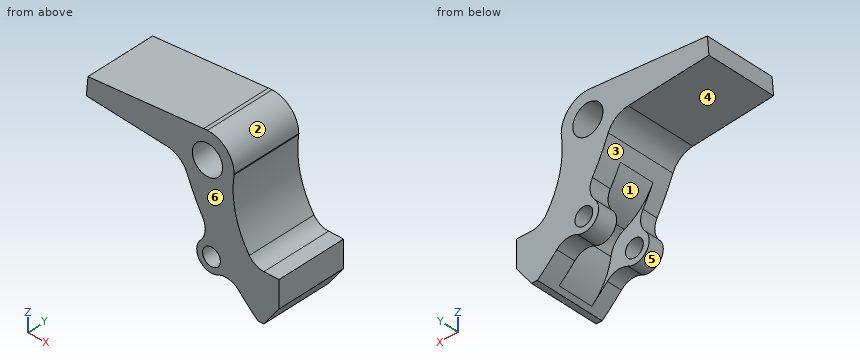
```python
from build123d import *

# Parameters (mm, degrees)
SKETCH1_R           = 2.55
SKETCH1_R_2         = 1.5
BOSS_EXTRUDE1_DEPTH = 11.9
SKETCH2_R           = 4
CUT_EXTRUDE1_DEPTH  = 3
FILLET1_R           = 10


with BuildPart() as part:
    # Sketch1 → Boss-Extrude1 (new body)
    with BuildSketch(Plane(origin=(0, 0, 0), x_dir=(1, 0, 0), z_dir=(0, 1, 0))):
        with BuildLine():
            Line((9.548719517, 20.446351577), (8.548719517, 20.439520648))
            ThreePointArc((8.548719517, 20.439520648), (6.873073378, 18.92667054), (5.279413844, 17.32768501))
            ThreePointArc((5.279413844, 17.32768501), (3.641729047, 16.438171118), (1.79479604, 16.687339585))
            ThreePointArc((1.79479604, 16.687339585), (-1.298720161, 15.927784086), (-1.135127046, 12.74658866))
            ThreePointArc((-1.135127046, 12.74658866), (-0.36458096, 11.049678177), (-0.744733852, 9.225197364))
            ThreePointArc((-0.744733852, 9.225197364), (-2.181853542, 6.500169129), (-3.4195031, 3.678943251))
            ThreePointArc((-3.4195031, 3.678943251), (-4.750151746, 1.944049699), (-6.794216917, 1.167983317))
            Line((-6.794216917, 1.167983317), (-20.434932532, -0.008444123))
            Line((-20.434932532, -0.008444123), (-20.171389856, -3.064230295))
            Line((-20.171389856, -3.064230295), (-0.61568325, -4.46265538))
            Line((-0.61568325, -4.46265538), (0.024630797, -4.508444123))
            ThreePointArc((0.024630797, -4.508444123), (3.206611312, -3.190424639), (4.524630797, -0.008444123))
            ThreePointArc((4.524630797, -0.008444123), (4.522964187, 0.074936031), (4.52153968, 0.158320674))
            ThreePointArc((4.52153968, 0.158320674), (4.763290961, 5.914837028), (7.103103866, 11.179929599))
            ThreePointArc((7.103103866, 11.179929599), (8.177074896, 12.128306877), (9.568395932, 12.47044575))
            Line((9.568395932, 12.47044575), (12.103260685, 12.47044575))
            Line((12.103260685, 12.47044575), (12.103260685, 16.957695738))
            Line((12.103260685, 16.957695738), (9.548719517, 20.446351577))
        make_face()
        with Locations(Location((0.024630797, -0.008444123, 0), (0, 0, 270))):
            Circle(SKETCH1_R, mode=Mode.SUBTRACT)
        with Locations(Location((0.707528049, 14.436151384, 0), (0, 0, 270))):
            Circle(SKETCH1_R_2, mode=Mode.SUBTRACT)
    extrude(amount=BOSS_EXTRUDE1_DEPTH)

    # Sketch2 → Cut-Extrude1 (cut, symmetric)
    with BuildSketch(Plane(origin=(0, 5.59, 0), x_dir=(1, 0, 0), z_dir=(0, 1, 0))):
        with Locations((0.707528049, 14.436151384)):
            Circle(SKETCH2_R)
    extrude(amount=CUT_EXTRUDE1_DEPTH, both=True, mode=Mode.SUBTRACT)

    # Fillet1
    # the kernel refuses this fillet: 10 mm, written as the material it takes off along each edge
    with BuildSketch(Plane(origin=(4.097372756, 8.59, -16.55958089), x_dir=(0.7539501243329342, 0, -0.6569316631266551), z_dir=(0, -1, 0))) as fillet1_piece_1:
        with BuildLine():
            CenterArc((5.165347529, 9.999376692), FILLET1_R, 229.371801611, 39.988476575)
            Line((-1.346130645, 2.409867354), (-1.997278462, 1.650916421))
            ThreePointArc((-1.997278462, 1.650916421), (-1.331632365, 0.837063937), (-0.987680479, -0.156484095))
            Line((-0.987680479, -0.156484095), (0.368749302, -0.929528887))
            ThreePointArc((0.368749302, -0.929528887), (1.299277263, -0.79792354), (5.042532309, -0.999937669))
            Line((5.042532309, -0.999937669), (5.053697329, 0))
        make_face()
    extrude(amount=6, mode=Mode.SUBTRACT)
    with BuildSketch(Plane(origin=(-0.34961624, 8.59, -10.578374051), x_dir=(-0.41195039334505656, 0, 0.9112062738056916), z_dir=(0, -1, 0))) as fillet1_piece_2:
        with BuildLine():
            CenterArc((5.165347529, -9.999376692), FILLET1_R, 90.639721814, 39.988476575)
            Line((-1.346130645, -2.409867354), (-1.997278462, -1.650916421))
            ThreePointArc((-1.997278462, -1.650916421), (-1.331632365, -0.837063937), (-0.987680479, 0.156484095))
            Line((-0.987680479, 0.156484095), (0.368749302, 0.929528887))
            ThreePointArc((0.368749302, 0.929528887), (1.299277263, 0.79792354), (5.042532309, 0.999937669))
            Line((5.042532309, 0.999937669), (5.053697329, 0))
        make_face()
    extrude(amount=6, mode=Mode.SUBTRACT)


solid = part.part
```
Read the model definition and answer for the solid it produces. Units are mm, in the model's axes. Face numbers are marked on the shaded views. A direction names the side the tool comes from. Give positions to 0.01 mm unless a question says otherwise; leave off trailing zeros. Write each loop counter-clockwise with the first axis right and the second up, starting at its lowest first coordinate (ties: lowest second). Pieces come first, ordered by that corner, then holes. Notation, with made-up numbers: (-16.75, 65) -> (-5.75, 65) arc R15 cw to (-5.75, 83) -> close; hole circle Ø11 at (39.5, 83.25). An arc over 180 degrees is marked (long way). Answer in a Markdown table with one row per item.
1) Section B-B on z = -15.25 is taken. Give the vertices of the cut face in (x, y), plus the area to 3 significant figures.
Results list:
| item | result |
|---|---|
| outline | (-1.66, 0) -> (-0.55, 0) -> (-0.55, 2.59) -> (-1.66, 2.59) -> close; (-1.66, 8.59) -> (-0.55, 8.59) -> (-0.55, 11.9) -> (-1.66, 11.9) -> close; (1.97, 0) -> (12.1, 0) -> (12.1, 11.9) -> (1.97, 11.9) -> (1.97, 8.59) -> (4.97, 8.59) -> (4.97, 2.59) -> (1.97, 2.59) -> close |
| area | 109 mm^2 |
2) Section C-C on y = 1.75 is taken. Give the vertices of the cut face in (x, z).
Results list:
| item | result |
|---|---|
| outline | (-20.43, 0.01) -> (-6.79, -1.17) arc R4 cw to (-3.42, -3.68) arc R42.86 ccw to (-0.74, -9.23) arc R3 cw to (-1.14, -12.75) arc R2.5 ccw to (1.79, -16.69) arc R3 cw to (5.28, -17.33) arc R42.86 ccw to (8.55, -20.44) -> (9.55, -20.45) -> (12.1, -16.96) -> (12.1, -12.47) -> (9.57, -12.47) arc R3 cw to (7.1, -11.18) arc R15.41 cw to (4.52, -0.16) arc R28.72 cw to (4.52, 0.01) arc R4.5 ccw to (0.02, 4.51) -> (-20.17, 3.06) -> close; hole circle Ø5.1 at (0.02, 0.01); hole circle Ø3 at (0.71, -14.44) |
3) Determine the mould class of the marked faces 4, 5 and 6 for opening direction Z: released by +Z, released by -Z, zero draft, split by the parting line, or undercut.
Results list:
| item | result |
|---|---|
| face 4 | released by -Z |
| face 5 | undercut |
| face 6 | zero draft |
4) Section A-A on y = 4.25 is taken. Give the vertices of the cut face in (x, z), plus the area to 3 significant figures.
Results list:
| item | result |
|---|---|
| outline | (-20.43, 0.01) -> (-6.79, -1.17) arc R4 cw to (-3.42, -3.68) arc R42.86 ccw to (-2.43, -5.97) arc R10 ccw to (2.4, -10.81) arc R4 cw to (4.67, -13.86) arc R10 ccw to (7.91, -19.88) arc R42.86 ccw to (8.55, -20.44) -> (9.55, -20.45) -> (12.1, -16.96) -> (12.1, -12.47) -> (9.57, -12.47) arc R3 cw to (7.1, -11.18) arc R15.41 cw to (4.52, -0.16) arc R28.72 cw to (4.52, 0.01) arc R4.5 ccw to (0.02, 4.51) -> (-20.17, 3.06) -> close; hole circle Ø5.1 at (0.02, 0.01) |
| area | 216 mm^2 |
5) A tool of negligible diameter and unlimited length cuts with its end or side. For the marked faces 1, 2 and 3, from which of +Z, -Z, +X, -X, +Y, -Y can it reach the whole face along a straight path? Write none if from no direction.
Results list:
| item | result |
|---|---|
| face 1 | -Z, -X |
| face 2 | +Z, +X, +Y, -Y |
| face 3 | -X, +Y, -Y |
6) Straight lines are drawn through the part: line 1 (Z direction, x = 2, y = 1); line 2 (X direction, y = 9, z = 0.5); line 3 (Y direction, x = 0.5, z = -11.25). For each, find the intervals that lie inside material, in ascending order. Write a range as [from, to].
Results list:
| item | result |
|---|---|
| line 1 | [-16.6, -15.2], [-13.67, -1.6], [1.62, 4.05] |
| line 2 | [-20.39, -2.48], [2.53, 4.5] |
| line 3 | [0, 2.59], [8.59, 11.9] |
7) Section D-D on z = 1 is taken. Give the vertices of the cut face in (x, y), plus the area to 3 significant figures.
Results list:
| item | result |
|---|---|
| outline | (-20.35, 0) -> (-2.32, 0) -> (-2.32, 11.9) -> (-20.35, 11.9) -> close; (2.37, 0) -> (4.41, 0) -> (4.41, 11.9) -> (2.37, 11.9) -> close |
| area | 239 mm^2 |
8) Each of these flat-tipped pins is pushed along its axis until it touches: pin 1 Ø2 at (x, y) = (-4, 2.5) entering from +Z; pin 2 Ø1 at (x, z) = (-2, -5.5) entering from -Y; pin 3 Ø3 at (x, z) = (0.02, 0.01) entering from -Y; pin 4 Ø4 at (y, z) = (3.5, -3.5) entering from +X. Where does it stop, or does it pass through?
Results list:
| item | result |
|---|---|
| pin 1 | z = 4.29 |
| pin 2 | y = 0 |
| pin 3 | through |
| pin 4 | x = 4.67 |
